Read the model definition and answer for the solid it produces. Units are mm, in the model's axes. A direction names the side the tool comes from. Round coordinates to 2 decimals unless told otherwise and drop trailing zeros. Loops run counter-clockwise (first coordinate to the right, second up) from the corner with the lowest first, then second, coordinate; pieces in that order, holes last. Notation, with made-up numbers: (76.25, 48) - (120.25, 48) arc R19 ccw to (120.25, 67) - close; hole circle Ø11 at (-13, 85). An arc over 180 degrees is marked (long way). Answer as CSV lines item,"result".
```python
from build123d import *

# Parameters (mm, degrees)
EXTRUDE_1_DEPTH           = 10
EXTRUDE_1_DEPTH_BACK      = 5
SKETCH_1_W                = 35
SKETCH_1_H                = 20
SKETCH_17_R               = 5
EXTRUDE_3_DEPTH           = 5
SKETCH_7_R                = 3
CUT_EXTRUDE_7_DEPTH       = 5
CUT_EXTRUDE_12_DEPTH      = 26.124689053
CUT_EXTRUDE_12_DEPTH_BACK = 26.124689053
EXTRUDE_2_DEPTH           = 15
SKETCH_19_R               = 22.5
SKETCH_19_R_2             = 20
EXTRUDE_4_DEPTH           = 6
SKETCH_20_R               = 2.5
SKETCH_20_R_2             = 1.5
CUT_EXTRUDE_16_DEPTH      = 6


with BuildPart() as part:
    # 草圖1 → 填料-伸長1 (new, two sides: drawn at the far end of the back side and taken through both)
    with BuildSketch(Plane(origin=(0, 0, 0), x_dir=(1, 0, 0), z_dir=(0, 1, 0)).offset(-EXTRUDE_1_DEPTH_BACK)):
        Rectangle(SKETCH_1_W, SKETCH_1_H)
    extrude(amount=EXTRUDE_1_DEPTH + EXTRUDE_1_DEPTH_BACK)

    # 草圖17 → 填料-伸長3 (add)
    with BuildSketch(Plane.XY.offset(10)):
        with Locations((10, 4.5)):
            Circle(SKETCH_17_R)
    extrude(amount=EXTRUDE_3_DEPTH)

    # 草圖7 → 除料-伸長7 (cut, symmetric)
    with BuildSketch(Plane.XY.offset(-10)):
        with Locations((10, 4.5)):
            Circle(SKETCH_7_R)
    extrude(amount=CUT_EXTRUDE_7_DEPTH, both=True, mode=Mode.SUBTRACT)

    # 草圖12 → 除料-伸長12 (cut, two sides: drawn at the far end of the back side and taken through both)
    with BuildSketch(Plane.XY.offset(-CUT_EXTRUDE_12_DEPTH_BACK)):
        with BuildLine():
            Line((15, 4.5), (15, -5))
            Line((15, -5), (17.54652099, -5))
            Line((17.54652099, -5), (17.54652099, 10.497831093))
            Line((17.54652099, 10.497831093), (5.54652099, 10.497831093))
            Line((5.54652099, 10.497831093), (5.54652099, 8.8762607))
            Line((5.54652099, 8.8762607), (7.581665389, 8.8762607))
            ThreePointArc((7.581665389, 8.8762607), (12.540504571, 8.806487725), (15, 4.5))
        make_face()
    extrude(amount=CUT_EXTRUDE_12_DEPTH + CUT_EXTRUDE_12_DEPTH_BACK, mode=Mode.SUBTRACT)

    # 草圖14 → 填料-伸長2 (add)
    with BuildSketch(Plane(origin=(0, -5, 0), x_dir=(1, 0, 0), z_dir=(0, 1, 0))):
        with BuildLine():
            Line((-17.5, 10), (-70.654637132, 58.47251336))
            ThreePointArc((-70.654637132, 58.47251336), (-111.24926813, 47.808473813), (-84.903421397, 15.135210044))
            Line((-84.903421397, 15.135210044), (-17.5, -10))
            Line((-17.5, -10), (-17.5, 10))
        make_face()
    extrude(amount=EXTRUDE_2_DEPTH)

    # 草圖19 → 填料-伸長4 (add)
    with BuildSketch(Plane(origin=(0, 10, 0), x_dir=(1, 0, 0), z_dir=(0, 1, 0))):
        with Locations(Location((-87.5, 40, 0), (0, 0, 90))):
            Circle(SKETCH_19_R)
        with Locations(Location((-87.5, 40, 0), (0, 0, 270))):
            Circle(SKETCH_19_R_2, mode=Mode.SUBTRACT)
    extrude(amount=EXTRUDE_4_DEPTH)

    # 草圖20 → 除料-伸長16 (cut)
    with BuildSketch(Plane(origin=(0, 10, 0), x_dir=(1, 0, 0), z_dir=(0, 1, 0))):
        with Locations(Location((-87.5, 48, 0), (0, 0, 270))):
            Circle(SKETCH_20_R)
        with Locations(Location((-87.5, 56.5, 0), (0, 0, 270))):
            Circle(SKETCH_20_R_2)
        with Locations(Location((-97, 40, 0), (0, 0, 270))):
            Circle(SKETCH_20_R)
        with Locations(Location((-104, 40, 0), (0, 0, 270))):
            Circle(SKETCH_20_R_2)
        with Locations(Location((-87.5, 32, 0), (0, 0, 90))):
            Circle(SKETCH_20_R)
        with Locations(Location((-87.5, 23.5, 0), (0, 0, 90))):
            Circle(SKETCH_20_R_2)
        with Locations(Location((-71, 40, 0), (0, 0, 90))):
            Circle(SKETCH_20_R_2)
        with Locations(Location((-78, 40, 0), (0, 0, 90))):
            Circle(SKETCH_20_R)
    extrude(amount=-CUT_EXTRUDE_16_DEPTH, mode=Mode.SUBTRACT)


solid = part.part
```
1) Find the intervals of material crossed by line 1 (X direction, y = 8.75, z = -40); line 2 (Y direction, x = -89.5, z = -58); line 3 (X direction, y = 6.5, z = -49), in increasing order.
Entries:
line 1,"x = -112.5 to -105.5, -102.5 to -99.5, -94.5 to -80.5, -75.5 to -72.5, -69.5 to -50.4"
line 2,"y = -5 to 10"
line 3,"x = -110.82 to -89.79, -85.21 to -60.27"
2) A cutting plane is placed at B-B, the plane z = -7.5. Determine the outline of the cut face in (x, y), plus the area to 3 significant figures.
Entries:
outline,"(-64.43, -5) - (15, -5) - (15, 4.5) arc R5 ccw to (7.58, 8.88) - (5.55, 8.88) - (5.55, 10) - (-64.43, 10) - close; hole circle Ø6 at (10, 4.5)"
area,"1,150 mm^2"
3) A cutting plane is placed at D-D, the plane x = -97. Determine the outline of the cut face in (y, z).
Entries:
outline,"(-5, -63.12) - (10, -63.12) - (10, -60.4) - (16, -60.4) - (16, -57.6) - (10, -57.6) - (10, -42.5) - (4, -42.5) - (4, -37.5) - (10, -37.5) - (10, -22.4) - (16, -22.4) - (16, -19.6) - (10, -19.6) - (10, -16.88) - (-5, -16.88) - close"
4) A tool of negligible diameter and unlimited length cuts with its end or side. For faces 1 (the face through (-88, 4, -32)), 2 (the face through (15, 0, 0)), 3 (the face through (12.39, 8.89, 5.1)), from which of +Z, -Z, +X, -X, +Y, -Y can it reach the whole face along a straight path? Write none if from no direction.
Entries:
face 1,"+Y"
face 2,"+Z, -Z, +X, +Y, -Y"
face 3,"+Z"
5) The mould has two halves that part along Z. Classify faces 4 (the face through (-1, 2, -10)), 5 (the face through (-88, 10, -40)), 6 (the face through (-45, 10, -19)): pulls with the +Z half, pulls with the -Z half, needs draft (parallel to the pull), parting line crosses it, or undercut.
Entries:
face 4,"pulls with the -Z half"
face 5,"undercut"
face 6,"needs draft"
6) A cutting plane is placed at A-A, the plane y = 13.25. Determine the outline of the cut face in (x, z), plus the area to 3 significant figures.
Entries:
outline,"circle Ø45 at (-87.5, -40); hole circle Ø40 at (-87.5, -40)"
area,"334 mm^2"
7) Each of these flat-tipped pins is pushed along its axis until it touches: P1, Ø2.5, axis at x = -104, z = -40, coming from the +Y side; P2, Ø3.5, axis at x = -104, z = -40, coming from the +Y side; P3, Ø1.5, axis at x = -85.5, y = 8, coming from the -Z side. Where does it stop, or does it pass through?
Entries:
P1,"stops at y = 4"
P2,"stops at y = 10"
P3,"stops at z = -64.97"
8) A cutting plane is placed at C-C, the plane y = -2.5. Determine the outline of the cut face in (x, z), plus the area to 3 significant figures.
Entries:
outline,"(-84.9, -15.14) arc R25 ccw (long way) to (-70.65, -58.47) - (-17.5, -10) - (15, -10) - (15, 10) - (-17.5, 10) - close"
area,"4,300 mm^2"
